Autodesk Inventor part; units mm, degrees
ref_plane "YZ Plane" through (0, 0, 0) normal (1, 0, 0) x (0, 1, 0)
ref_plane "XZ Plane" through (0, 0, 0) normal (0, 1, 0) x (-1, 0, 0)
ref_plane "XY Plane" through (0, 0, 0) normal (0, 0, 1) x (1, 0, 0)
sketch "Szkic1" plane through (0, 0, 0) normal (0, 0, 1) x (1, 0, 0)
  circle A0 centre (-13.3747, 0.2773) radius 22.5
  circle A1 centre (38.6246, 0.0082) radius 13
  line L0 (8.9598, 3.0013) -> (25.9772, 3.0013)
  line L1 (25.9772, 3.0013) -> (25.9772, -2.9987)
  line L2 (25.9772, -2.9987) -> (8.9598, -2.9987)
  line L3 (8.9598, -2.9987) -> (8.9598, 3.0013)
  line L4 (25.9772, 3.0013) -> (8.9598, -2.9987) construction
  line L5 (1.1462, -22.2227) -> (1.1462, -37.7227)
  line L6 (1.1462, -37.7227) -> (-28.8538, -37.7227)
  line L7 (-28.8538, -37.7227) -> (-28.8538, -22.2227)
  line L8 (-28.8538, -22.2227) -> (-28.8538, -16.052)
  line L9 (1.1462, -22.2227) -> (1.1462, -16.9097)
  point P0 (0, 0)
  point P1 (17.4685, 0.0013)
  point P2 (-13.8538, -22.2176)
  point P3 (8.9598, -2.4467)
  point P4 (25.9739, 3.0013)
  dimension "d1" = 26
  dimension "d0" = 45
  dimension "d2" = 52
  dimension "d3" = 6
  dimension "d4" = 30
  dimension "d5" = 38
extrude "Wyciągnięcie proste1" add sketch "Szkic1" along normal mid plane 20
sketch "Szkic2" plane through (0, 0, 10) normal (0, 0, 1) x (1, 0, 0)
  point P0 (0, 0)
sketch "Szkic3" plane through (8.9598, 3.0013, 10) normal (0, 1, 0) x (1, 0, 0)
  line L0 (29.8394, 10) -> (-7.8136, 10)
  line L1 (-7.8136, 20) -> (-7.8136, 0)
  line L2 (-7.8136, 13) -> (29.8394, 13)
  line L3 (29.8394, 13) -> (29.8394, 7)
  line L4 (29.8394, 7) -> (-7.8136, 7)
  line L5 (-7.8136, 7) -> (-7.8136, 13)
  line L6 (-7.8136, 13) -> (29.8394, 7) construction
  line L7 (29.8394, 13) -> (-7.8136, 7) construction
  point P0 (-8.9598, 10)
  point P1 (11.0129, 10)
  dimension "d8" = 6
extrude "Wyciągnięcie proste2" add sketch "Szkic3" along normal blind 10 and the other way blind 16
sketch "Szkic4" plane through (0, 0, 10) normal (0, 0, 1) x (1, 0, 0)
  arc A0 (8.9598, 3.0013) -> (-28.8538, -16.052) centre (-13.3747, 0.2773) ccw
  arc A1 (25.9772, -2.9987) -> (25.9739, 3.0013) centre (38.6246, 0.0082) ccw
  point P0 (0, 0)
sketch "Szkic5" plane through (0, 0, 10) normal (0, 0, 1) x (1, 0, 0)
  line L0 (-12.3538, -38.025) -> (-15.3538, -38.025)
  line L1 (-15.3538, -38.025) -> (-15.3538, -14.6448)
  line L2 (-15.3538, -14.6448) -> (-12.3538, -14.6448)
  line L3 (-12.3538, -14.6448) -> (-12.3538, -38.025)
  line L4 (-12.3538, -38.025) -> (-15.3538, -14.6448) construction
  line L5 (-15.3538, -38.025) -> (-12.3538, -14.6448) construction
  point P0 (0, 0)
  point P1 (-13.8538, -26.3349)
  dimension "d13" = 3
hole "Otwór1" at (-13.3747, 0.2773, 10) direction (0, 0, -1) diameter 32 end through all
sketch "Szkic6" plane through (0, 0, 10) normal (0, 0, 1) x (1, 0, 0)
  arc A0 (25.9772, -2.9987) -> (25.9739, 3.0013) centre (38.6246, 0.0082) ccw
  point P0 (0, 0)
hole "Otwór2" at (38.6246, 0.0082, 10) direction (0, 0, -1) diameter 14 end through all
extrude "Wyciągnięcie proste3" cut sketch "Szkic5" against normal through all
sketch "Szkic7" plane through (1.1462, -37.7227, 10) normal (1, 0, 0) x (0, 0, -1)
  point P0 (10, 37.7227)
  point P1 (10, 11.5)
hole "Otwór3" at (1.1462, -26.2227, 0) direction (-1, 0, 0) diameter 8 end through all
The model under review builds one solid part; all positions refer to its coordinate system, in mm. A direction names the side the tool comes from. Give positions to 0.01 mm unless a question says otherwise; leave off trailing zeros. Write each loop counter-clockwise with the first axis right and the second up, starting at its lowest first coordinate (ties: lowest second). Pieces come first, ordered by that corner, then holes. Notation, with made-up numbers: (74.5, 83) -> (130.5, 83) arc R13 ccw to (130.5, 108) -> close; hole circle Ø7 at (72.5, 66). An arc over 180 degrees is marked (long way). Put each result on its own line as item: value.
(1) For pin 1 Ø7 at (y, z) = (-26.22, 0) entering from -X; pin 2 Ø10 at (y, z) = (-29, 0.5) entering from -X; pin 3 Ø2 at (x, z) = (6.5, -7) entering from -Y; pin 4 Ø5 at (y, z) = (2, -3.5) entering from +X, all flat-tipped, find the tip position at first contact; note any pin that passes through.
Results are:
pin 1: through
pin 2: x = -28.85
pin 3: y = -11.97
pin 4: x = 51.62
(2) We need section A-A, the plane x = -11. Give the boundary of the cut face in (y, z).
Results are:
outline: (-37.72, -10) -> (-15.55, -10) -> (-15.55, 10) -> (-37.72, 10) -> close; (16.1, -10) -> (22.65, -10) -> (22.65, 10) -> (16.1, 10) -> close; hole circle Ø8 at (-26.22, 0)
(3) The part is to be moulded in two halves that separate along Z. For faces 4 (the flat face through (1, -10, -10)), 5 (the flat face through (18, 8, 3)), 6 (the flat face through (22, -12.999, 0)), 7 (the cylindrical face through (-5.7, -30.19, 0.52)), say which applies: pulls with the +Z half, pulls with the -Z half, needs draft (parallel to the pull), parting line crosses it, or undercut.
Results are:
face 4: pulls with the -Z half
face 5: pulls with the +Z half
face 6: needs draft
face 7: undercut
(4) To check wall thickness, follow probe 1 along X at (y, z) = (-22.5, -4.25); probe 2 along Y at (x, z) = (-6.5, 0); probe 3 along Y at (x, z) = (17, 8.25). State the ranges of each line that lie inside material, in increasing order. Write a range as from..to.
Results are:
probe 1: -28.85..-15.35, -12.35..1.15
probe 2: -37.72..-30.22, -22.22..-14.17, 14.73..21.7
probe 3: -3..3
(5) Tool access review of faces 1 (the flat face through (17, 3.001, 6)), 2 (the cylindrical face through (51.614, 0.545, -0.14)), 3 (the flat face through (18, 8, -3)): name each direction out of +Z, -Z, +X, -X, +Y, -Y from which nothing blocks a thin tool from reaching the whole face with its end or side.
Results are:
face 1: +Z, +Y
face 2: none
face 3: -Z, +Y
(6) We need section C-C, the plane y = -10. Give the boundary of the cut face in (x, z).
Results are:
outline: (-33.39, -10) -> (-25.64, -10) -> (-25.64, 10) -> (-33.39, 10) -> close; (-1.11, -10) -> (6.64, -10) -> (6.64, -3) -> (30.33, -3) -> (30.33, -10) -> (46.92, -10) -> (46.92, 10) -> (30.33, 10) -> (30.33, 3) -> (6.64, 3) -> (6.64, 10) -> (-1.11, 10) -> close
(7) We need section D-D, the plane x = 40. Give the boundary of the cut face in (y, z).
Results are:
outline: (-12.92, -10) -> (-6.86, -10) -> (-6.86, 10) -> (-12.92, 10) -> close; (6.87, -10) -> (12.94, -10) -> (12.94, 10) -> (6.87, 10) -> close
(8) We need section B-B, the plane z = 0.5. State how many separate pieces and enclosed holes the cut face has, and give its area (3 significant figures).
Results are:
separate pieces: 3
enclosed holes: 1
area: 1,940 mm²
